Check sheet for the modelled part. Datum: model origin and axes. Units: mm. A direction names the side the tool comes from. Round coordinates to 2 decimals unless told otherwise and drop trailing zeros. Write each loop counter-clockwise with the first axis right and the second up, starting at its lowest first coordinate (ties: lowest second). Pieces come first, ordered by that corner, then holes.
Item 1: Section check D-D, the plane z = -5.5. Record the cut outline in (x, y), plus the area to 3 significant figures.
Item 2: Section check C-C, the plane x = 3.5. Record the cut outline in (y, z), plus the area to 3 significant figures.
Item 3: Set-up check for faces 1 (the cylindrical face through (11, -5, 19)), 2 (the cylindrical face through (-20.9, 0.6, -0.3)): record each of +Z, -Z, +X, -X, +Y, -Y from which the full face is reachable in a straight line by a thin tool's end or side.
Item 4: Release check for a two-part mould opening along Z. For faces 3 (the flat face through (-1, -10, -1)), 4 (the flat face through (-9, 13.5, -29)) record: pulls with the +Z half, pulls with the -Z half, needs draft (parallel to the pull), parting line crosses it, or undercut.
Item 5: Section check B-B, the plane z = 11. Record the cut outline in (x, y), plus the area to 3 significant figures.
Item 6: Depth check by flat-ended pin: pin 1 (3 mm diameter, centred on x = -13.5, z = 3.5, fed in from +Y); pin 2 (1.7 mm diameter, centred on x = 20, z = 0, fed in from +Y); pin 3 (16 mm diameter, centred on x = -11.5, z = -4.5, fed in from +Y). Enter the tip coordinate at first touch or a pass-through.
Item 7: Section check A-A, the plane y = 5.25. State how many separate pieces and enclosed holes the cut face has, plus the area to 3 significant figures.
Item 8: Material ranges on line 1 along Z through (x, y) = (1, 6.75); line 2 along X through (y, z) = (-6.5, 0.5); line 3 along Y through (x, z) = (-22, -9.5), recorded low to high.
Autodesk Fusion 360 part; units mm, degrees
sketch "BaseSketch" plane through (0, 0, 0) normal (0, 1, 0) x (1, 0, 0)
  circle A0 centre (0, 0) radius 38.5
  circle A1 centre (0, 0) radius 26.5
  dimension "d1" = 77
  dimension "d2" = 53
extrude "Extrude1" add sketch "BaseSketch" against normal blind 10 contours A0 | A1
extrude "Extrude2" add sketch "BaseSketch" along normal blind 15
sketch "ORingSketch" plane through (0, 15, 0) normal (0, 1, 0) x (-1, 0, 0)
  circle A0 centre (0, 0) radius 26.5
  circle A1 centre (0, 0) radius 38.5
  circle A2 centre (0, 0) radius 30
  circle A3 centre (0, 0) radius 32.5
  dimension "d10" = 60
  dimension "d11" = 65
extrude "Extrude3" cut sketch "ORingSketch" against normal blind 1.5 contours A3
sketch "ScrewSketch" plane through (0, 15, 0) normal (0, 1, 0) x (-1, 0, 0)
  circle A0 centre (0, 0) radius 38.5
  circle A1 centre (0, 0) radius 32.5
  circle A2 centre (-35.5, 0) radius 0.95
  circle A3 centre (-25.1023, -25.1023) radius 0.95
  circle A4 centre (0, -35.5) radius 0.95
  circle A5 centre (25.1023, -25.1023) radius 0.95
  circle A6 centre (35.5, 0) radius 0.95
  circle A7 centre (25.1023, 25.1023) radius 0.95
  circle A8 centre (0, 35.5) radius 0.95
  circle A9 centre (-25.1023, 25.1023) radius 0.95
  dimension "d16" = 1.9
  dimension "d19" = 360
  dimension "d22" = 35.5
extrude "Extrude4" cut sketch "ScrewSketch" against normal blind 15 contours A2 | A3 | A4 | A5 | A6 | A7 | A8 | A9
sketch "StandoffSketch" plane through (0, 0, 0) normal (0, 1, 0) x (-1, 0, 0)
  circle A0 centre (0, 0) radius 26.5
  circle A1 centre (0, 0) radius 25
  circle A2 centre (-20, 0) radius 0.95
  circle A3 centre (-20, 0) radius 2.45
  circle A4 centre (0, -20) radius 0.95
  circle A5 centre (0, -20) radius 2.45
  circle A6 centre (20, 0) radius 0.95
  circle A7 centre (20, 0) radius 2.45
  circle A8 centre (0, 20) radius 0.95
  circle A9 centre (0, 20) radius 2.45
  dimension "d25" = 50
  dimension "d27" = 1.9
  dimension "d28" = 20
  dimension "d29" = 4.9
  dimension "d31" = 360
extrude "Extrude5" add sketch "StandoffSketch" along normal blind 8.5 contours A3 | A5 | A7 | A9
extrude "Extrude6" cut sketch "StandoffSketch" against normal blind 7 contours A2 | A4 | A6 | A8
ref_plane "WorkPlane1" through (0, 15, 0) normal (0, 1, 0) x (1, 0, 0)
sketch "RubberPlugSketch" plane through (0, 0, 0) normal (0, 1, 0) x (-1, 0, 0)
  circle A0 centre (20, 0) radius 2.45
  circle A1 centre (0, -20) radius 2.45
  circle A2 centre (0, 0) radius 26.5
  circle A3 centre (-20, 0) radius 2.45
  circle A4 centre (0, 20) radius 2.45
  circle A5 centre (-13.9903, 13.5103) radius 6.25
  line L0 (0, 0) -> (-26.5, 0) construction
  line L1 (0, 0) -> (-13.9903, 13.5103) construction
  dimension "d37" = 12.5
  dimension "d38" = 19.4488
  dimension "d39" = 44
extrude "Extrude7" cut sketch "RubberPlugSketch" against normal blind 10 contours A5
equation "d1 = diameter"
equation "d2 = PCBdiameter + tolerance"
equation "tolerance = 3 mm"
equation "CaseBottomThick = 10 mm"
equation "height = 25 mm"
equation "d8 = height - CaseBottomThick"
equation "d10 = d11 - 5 mm"
equation "diameter = 77 mm"
equation "screwDiameter = 1.9 mm"
equation "d16 = screwDiameter"
equation "screwDepth = 15 mm"
equation "d22 = diameter / 2 - 3 mm"
equation "d25 = PCBdiameter"
equation "PCBdiameter = 50 mm"
equation "d27 = screwDiameter"
equation "d28 = PCBdiameter / 2 - 5 mm"
equation "d29 = screwDiameter + tolerance"
equation "d32 = 5.5 mm + tolerance"
Values found:
1. outline: (-38.11, -10) - (38.11, -10) - (38.11, 15) - (32.03, 15) - (32.03, 13.5) - (29.49, 13.5) - (29.49, 15) - (25.92, 15) - (25.92, 0) - (-25.92, 0) - (-25.92, 15) - (-29.49, 15) - (-29.49, 13.5) - (-32.03, 13.5) - (-32.03, 15) - (-38.11, 15) - close
1. area: 1,120 mm2
2. outline: (-10, -38.34) - (15, -38.34) - (15, -32.31) - (13.5, -32.31) - (13.5, -29.8) - (15, -29.8) - (15, -26.27) - (0, -26.27) - (0, 26.27) - (15, 26.27) - (15, 29.8) - (13.5, 29.8) - (13.5, 32.31) - (15, 32.31) - (15, 38.34) - (-10, 38.34) - close
2. area: 1,120 mm2
3. face 1: +Y, -Y
3. face 2: +Y
4. face 3: needs draft
4. face 4: undercut
5. outline: (-36.9, -10) - (8.27, -10) - (8.27, 0) - (-24.11, 0) - (-24.11, 15) - (-27.91, 15) - (-27.91, 13.5) - (-30.58, 13.5) - (-30.58, 15) - (-36.9, 15) - close; (19.71, -10) - (36.9, -10) - (36.9, 15) - (30.58, 15) - (30.58, 13.5) - (27.91, 13.5) - (27.91, 15) - (24.11, 15) - (24.11, 0) - (19.71, 0) - close
5. area: 999 mm2
6. pin 1: stops at y = 0
6. pin 2: stops at y = -7
6. pin 3: stops at y = 8.5
7. separate pieces: 5
7. enclosed holes: 13
7. area: 2,490 mm2
8. line 1: z = -38.49 to -26.48, -22.24 to -17.76, 17.76 to 22.24, 26.48 to 38.49
8. line 2: x = -38.5 to -20.81, -19.19 to 19.19, 20.81 to 38.5
8. line 3: y = -10 to 0
